Geometry check sheet. Reference: drawing and pictorial views, mm from the part's lowest x, y, z. Round coordinates to 2 decimals unless told otherwise and drop trailing zeros. Loops run counter-clockwise (first coordinate to the right, second up) from the corner with the lowest first, then second, coordinate; pieces in that order, holes last. Notation, with made-up numbers: (-3.75, -27) - (33.25, -27) arc R25 ccw to (33.25, -9) - close; hole circle Ø6 at (21.25, 57). An arc over 180 degrees is marked (long way). Return JSON: item names as keys, results as strings.
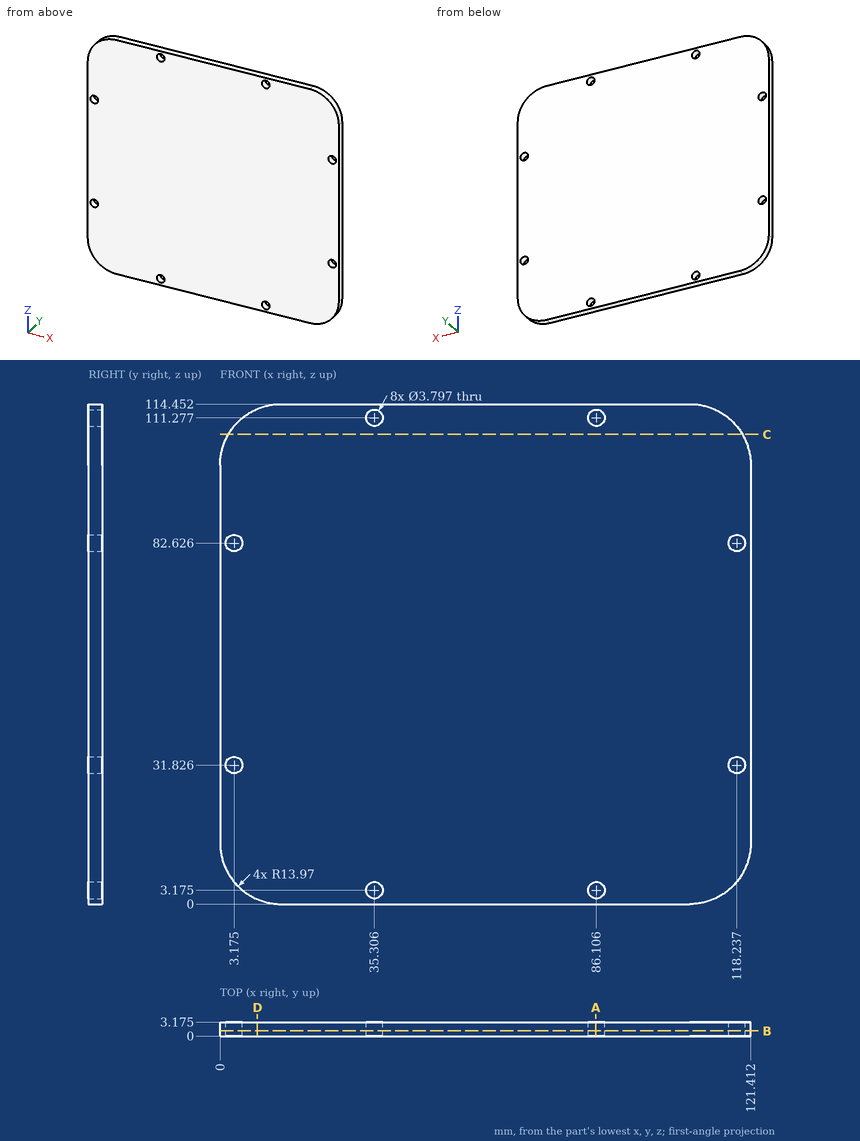
Q1. Sectioned sample at C-C (z = 107.5). Enter the section's corners in (x, y) (1 decimal).
Answer key:
{"outline": "(1.9, 0) - (119.5, 0) - (119.5, 3.2) - (1.9, 3.2) - close"}
Q2. Sectioned sample at D-D (x = 8.5). Enter the section's corners in (y, z) (1 decimal).
Answer key:
{"outline": "(0, 1.1) - (3.2, 1.1) - (3.2, 113.3) - (0, 113.3) - close"}
Q3. Sectioned sample at B-B (y = 1.15). State how many separate pieces and enclosed holes the cut face has, plus the area to 3 significant figures.
Answer key:
{"separate pieces": "1", "enclosed holes": "8", "area": "13,600 mm²"}
Q4. Scan lines: probe 1 along X at (y, z) = (1.3, 82) (1 decimal); probe 2 along X at (y, z) = (2.4, 101.5) (1 decimal); probe 3 along X at (y, z) = (2.5, 105). Record each from-to range of solid material in increasing order. Write a range as [from, to].
Answer key:
{"probe 1": "x = [0, 1.4], [5, 116.4], [120, 121.4]", "probe 2": "x = [0, 121.4]", "probe 3": "x = [0.75, 120.66]"}
Q5. Depth check by flat-ended pin: P1, Ø4, axis at x = 64.5, z = 38, coming from the -Y side. Enter the tip coordinate at first touch or a pass-through.
Answer key:
{"P1": "stops at y = 0"}
Q6. Sectioned sample at A-A (x = 86). Enter the section's corners in (y, z) (1 decimal).
Answer key:
{"outline": "(0, 0) - (3.2, 0) - (3.2, 1.3) - (0, 1.3) - close; (0, 5.1) - (3.2, 5.1) - (3.2, 109.4) - (0, 109.4) - close; (0, 113.2) - (3.2, 113.2) - (3.2, 114.5) - (0, 114.5) - close"}
